Here's how the part is built. I have some questions about the finished solid (model axes, mm). Face numbers are marked on the shaded views. Coordinates: 2 decimals unless noted, no trailing zeros. Write each loop counter-clockwise with the first axis right and the second up, starting at its lowest first coordinate (ties: lowest second). Pieces come first, ordered by that corner, then holes. Notation, with made-up numbers: M 9,21 L 36,21 A32 ccw 36,56 Z; hole C 71,44 d10. An arc over 180 degrees is marked long. Use a Markdown table: item, result.
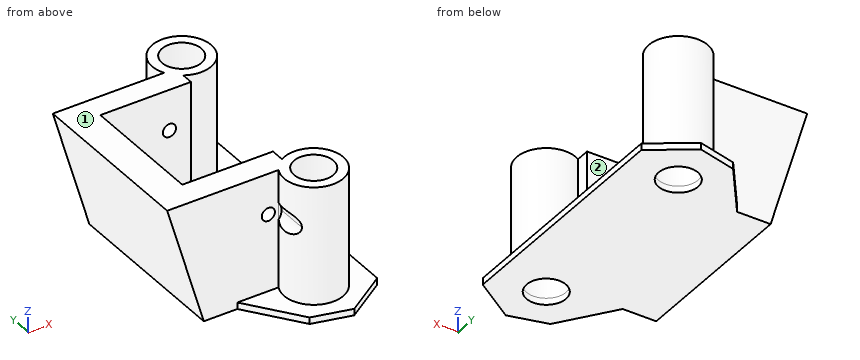
```python
from build123d import *

# Parameters (mm, degrees)
CYLINDER001_R           = 2
CYLINDER001_DEPTH       = 10
CYLINDER_R              = 2
CYLINDER_DEPTH          = 10
PAD007_DEPTH            = 17
SKETCH002_W             = 19
SKETCH002_H             = 19
PAD002_DEPTH            = 11
SKETCH003_R             = 1
PAD003_DEPTH            = 27
PAD003_FACE5_W          = 19
PAD003_FACE5_H          = 19
PAD004_DEPTH            = 24
BODY001_PLACEMENT_ANGLE = 159.7
SKETCH_R                = 3
PAD_DEPTH               = 1
SKETCH001_R             = 4.5
PAD001_DEPTH            = 18
PAD001_FACE25_R         = 3
POCKET_DEPTH            = 22
POCKET_FACE26_R         = 3
POCKET001_DEPTH         = 31
POCKET001_FACE18_W      = 13.265998
POCKET001_FACE18_H      = 18
PAD005_DEPTH            = 8
PAD005_FACE17_W         = 13.265998
PAD005_FACE17_H         = 18
PAD006_DEPTH            = 8


with BuildPart() as cylinder001:
    # Cylinder001 → Cylinder001 (new body)
    with BuildSketch(Plane(origin=(43.8, 13.3, 12.7), x_dir=(-1, 0, 0), z_dir=(0, 1, 0))):
        Circle(CYLINDER001_R)
    extrude(amount=CYLINDER001_DEPTH)


with BuildPart() as cylinder:
    # Cylinder → Cylinder (new body)
    with BuildSketch(Plane(origin=(43.8, -13.3, 12.7), x_dir=(1, 0, 0), z_dir=(0, -1, 0))):
        Circle(CYLINDER_R)
    extrude(amount=CYLINDER_DEPTH)


with BuildPart() as body002:
    # Sketch005 → Pad007 (new body, symmetric)
    with BuildSketch(Plane.XZ):
        Polygon((21.007471, 20.364401), (29.359247, -8.113389), (3.411231, -3.850644), (-10.027989, 26.995327), align=None)
    extrude(amount=PAD007_DEPTH, both=True)


with BuildPart() as body002_1:
    # Body002 placement: moved
    add(body002.part.moved(Location((7, 0, 0))))


with BuildPart() as body001:
    # Sketch002 → Pad002 (new body)
    with BuildSketch(Plane.YZ):
        with Locations((0.156277, 39.976883)):
            Rectangle(SKETCH002_W, SKETCH002_H)
    extrude(amount=PAD002_DEPTH)

    # Sketch003 (on Face2 of Pad002) → Pad003 (join, symmetric)
    with BuildSketch(Plane.ZX.offset(9.656277)):
        with Locations((39.976883, 0)):
            Circle(SKETCH003_R)
    extrude(amount=PAD003_DEPTH, both=True)

    # Pad003 Face5 → Pad004 (add)
    with BuildSketch(Plane(origin=(11, 0.156277, 39.976883), x_dir=(0, -1, 0), z_dir=(1, 0, 0))):
        Rectangle(PAD003_FACE5_W, PAD003_FACE5_H)
    extrude(amount=-PAD004_DEPTH)


with BuildPart() as body001_1:
    # Body001 placement: moved
    add(body001.part.moved(Location((29.937834, 0, 50.257929))).rotate(Axis((29.937834, 0, 50.257929), (0, 1, 0)), BODY001_PLACEMENT_ANGLE))


with BuildPart() as cut003:
    # Sketch → Pad (new body)
    with BuildSketch(Plane.XY):
        Polygon((61.12867, 22.644966), (55.288719, 21.173481), (49.485474, 13.265998), (24.71945, 13.265998), (24.71945, 0), (24.71945, -13.265998), (49.485474, -13.265998), (55.288719, -21.173481), (61.12867, -22.644966), (67.424286, -18.389174), (67.424286, 0), (67.424286, 18.389174), align=None)
        with Locations((59.784004, 15.3)):
            Circle(SKETCH_R, mode=Mode.SUBTRACT)
        with Locations((59.784004, -15.3)):
            Circle(SKETCH_R, mode=Mode.SUBTRACT)
    extrude(amount=PAD_DEPTH)

    # Sketch001 (on Face16 of Pad) → Pad001 (join)
    with BuildSketch(Plane.XY.offset(1)):
        with Locations((59.784004, 15.3)):
            Circle(SKETCH001_R)
        with Locations((59.784004, -15.3)):
            Circle(SKETCH001_R)
        Polygon((24.71945, 0), (24.71945, 13.265998), (49.485474, 13.265998), (49.485474, 0), (49.485474, -13.265998), (24.71945, -13.265998), align=None)
    extrude(amount=PAD001_DEPTH)

    # Pad001 Face25 → Pocket (cut)
    with BuildSketch(Plane(origin=(59.784004, -15.3, 1), x_dir=(0, -1, 0), z_dir=(0, 0, -1))):
        Circle(PAD001_FACE25_R)
    extrude(amount=-POCKET_DEPTH, mode=Mode.SUBTRACT)

    # Pocket Face26 → Pocket001 (cut)
    with BuildSketch(Plane(origin=(59.784004, 15.3, 1), x_dir=(0, -1, 0), z_dir=(0, 0, -1))):
        Circle(POCKET_FACE26_R)
    extrude(amount=-POCKET001_DEPTH, mode=Mode.SUBTRACT)

    # Pocket001 Face18 → Pad005 (add)
    with BuildSketch(Plane(origin=(49.485474, 6.632999, 10), x_dir=(0, -1, 0), z_dir=(1, 0, 0))):
        Rectangle(POCKET001_FACE18_W, POCKET001_FACE18_H)
    extrude(amount=PAD005_DEPTH)

    # Pad005 Face17 → Pad006 (add)
    with BuildSketch(Plane(origin=(49.485474, -6.632999, 10), x_dir=(0, -1, 0), z_dir=(1, 0, 0))):
        Rectangle(PAD005_FACE17_W, PAD005_FACE17_H)
    extrude(amount=PAD006_DEPTH)


with BuildPart() as cut003_1:
    # Body placement: moved
    add(cut003.part.moved(Location((-10.4, 0, 0))))

    # Cut: cut Body001
    add(body001_1.part, mode=Mode.SUBTRACT)

    # Cut001: cut Body002
    add(body002_1.part, mode=Mode.SUBTRACT)

    # Cut002: cut Cylinder
    add(cylinder.part, mode=Mode.SUBTRACT)

    # Cut003: cut Cylinder001
    add(cylinder001.part, mode=Mode.SUBTRACT)


solid = cut003_1.part
```
1. Suppose I cut it at B-B on z = 8.75. Write out the boundary of the cut face in (x, y).
Answers follow:
| item | result |
|---|---|
| outline | M 31.41,-13.27 L 45.37,-13.27 A4.5 ccw long 47.09,-11.43 L 47.09,-9.34 L 33.56,-9.34 L 33.56,9.66 L 47.09,9.66 L 47.09,11.43 A4.5 ccw long 45.37,13.27 L 31.41,13.27 Z; hole C 49.38,-15.3 d6; hole C 49.38,15.3 d6 |
2. I need wall thicknesses on probe 1 along Y at (x, z) = (42.5, 17); probe 2 along X at (y, z) = (-15.3, 8.25); probe 3 along Y at (x, z) = (47, 13.5). Which ranges of each line are inside material? Lowest first, please.
Answers follow:
| item | result |
|---|---|
| probe 1 | y = -13.27 to -9.34, 9.66 to 13.27 |
| probe 2 | x = 44.88 to 46.38, 52.38 to 53.88 |
| probe 3 | y = -19.12 to -17.12, -13.48 to -9.34, 9.66 to 13.48, 17.12 to 19.12 |
3. Suppose I cut it at D-D on z = 1.75. Write out the boundary of the cut face in (x, y).
Answers follow:
| item | result |
|---|---|
| outline | M 33.47,-13.27 L 45.37,-13.27 A4.5 ccw long 47.09,-11.43 L 47.09,11.43 A4.5 ccw long 45.37,13.27 L 33.47,13.27 Z; hole M 36.15,-9.34 L 41.41,-9.34 L 41.41,9.66 L 36.15,9.66 Z; hole C 49.38,-15.3 d6; hole C 49.38,15.3 d6 |
4. Will these pins go through, and if not, where does the flat tip stop? pin 1 Ø0.5 at (x, z) = (45.5, 12.5) entering from +Y; pin 2 Ø8.5 at (x, z) = (40.5, 8.5) entering from -Y; pin 3 Ø3 at (x, z) = (47, 9) entering from +Y.
Answers follow:
| item | result |
|---|---|
| pin 1 | stops at y = 13.3 |
| pin 2 | stops at y = -13.27 |
| pin 3 | stops at y = 19.71 |
5. Suppose I cut it at C-C on x = 31.25. Write out the boundary of the cut face in (y, z), and give its area (3 significant figures).
Answers follow:
| item | result |
|---|---|
| outline | M -13.27,9.31 L 13.27,9.31 L 13.27,19 L -13.27,19 Z; hole M -9.34,15 L 9.66,15 L 9.66,18.25 L -9.34,18.25 Z |
| area | 196 mm2 |
6. Suppose I cut it at A-A on y = -15.3. Write out the boundary of the cut face in (x, z).
Answers follow:
| item | result |
|---|---|
| outline | M 40.58,0 L 46.38,0 L 46.38,19 L 44.88,19 L 44.88,14.38 A2 cw 44.88,11.02 L 44.88,1 L 40.58,1 Z; M 52.38,0 L 57.02,0 L 57.02,1 L 53.88,1 L 53.88,19 L 52.38,19 Z |
7. We'd pull the mould along Y, two halves only. Please class the marked faces 1 and 2: +Y half, -Y half, draft (parallel to the pull), parting line (faces both ways), or undercut.
Answers follow:
| item | result |
|---|---|
| face 1 | draft |
| face 2 | undercut |
